from build123d import *

# Parameters (mm, degrees)
F1_DEPTH  = 25
F2_R      = 7.65
F3_DEPTH  = 1
F5_DEPTH  = 11
F7_W      = 10
F7_H      = 20
F10_W     = 10
F10_H     = 11
F13_START = -10
F13_DEPTH = 14
F14_START = -34
F14_DEPTH = 14
F15_R     = 5
F16_DEPTH = 7


with BuildPart() as f1:
    # F0 (on Top) → F1 (new body)
    with BuildSketch(Plane.XY):
        with BuildLine():
            ThreePointArc((0, 2), (0.5857864376, 0.5857864376), (2, 0))
            Line((2, 0), (116, 0))
            ThreePointArc((116, 0), (117.4142135624, 0.5857864376), (118, 2))
            Line((118, 2), (118, 98))
            ThreePointArc((118, 98), (117.4142135624, 99.4142135624), (116, 100))
            Line((116, 100), (2, 100))
            ThreePointArc((2, 100), (0.5857864376, 99.4142135624), (0, 98))
            Line((0, 98), (0, 2))
        make_face()
    extrude(amount=F1_DEPTH)

    # F2 (on face) → F3 (join)
    with BuildSketch(Plane.XY.offset(25)):
        with Locations((35, 28)):
            Circle(F2_R)
        with BuildLine():
            Line((23.7, 25.7), (23.7, 30.3))
            ThreePointArc((23.7, 30.3), (15, 39), (6.3, 30.3))
            Line((6.3, 30.3), (6.3, 25.7))
            ThreePointArc((6.3, 25.7), (15, 17), (23.7, 25.7))
        make_face()
        with Locations((53, 28)):
            Circle(F2_R)
    extrude(amount=F3_DEPTH)

    # F4 (on face) → F5 (cut)
    with BuildSketch(Plane.XY.offset(26)):
        Polygon((20.75, 25), (20.75, 31), (18.5, 31), (18.5, 34), (11.5, 34), (11.5, 31), (9.25, 31), (9.25, 25), (11.5, 25), (11.5, 22), (18.5, 22), (18.5, 25), align=None)
    extrude(amount=-F5_DEPTH, mode=Mode.SUBTRACT)

    # F7 (on offset) → F8 (revolve, cut)
    with BuildSketch(Plane.XY.offset(30)):
        with Locations((15, 80)):
            Rectangle(F7_W, F7_H)
        with Locations((35, 80)):
            Rectangle(F7_W, F7_H)
    revolve(axis=Axis((25, 70, 30), (1, 0, 0)), mode=Mode.SUBTRACT)

    # F10 (on offset) → F11 (revolve, cut)
    with BuildSketch(Plane.XY.offset(27)):
        with Locations((55, 55.5)):
            Rectangle(F10_W, F10_H)
    revolve(axis=Axis((55, 61, 27), (1, 0, 0)), mode=Mode.SUBTRACT)

    # F12 (on face) → F13 (cut)
    with BuildSketch(Plane.YZ.offset(118).offset(F13_START)):
        with BuildLine():
            Line((42, 1), (57, 1))
            ThreePointArc((57, 1), (92.8019763155, 40.7707415594), (49.5, 72.2100837829))
            ThreePointArc((49.5, 72.2100837829), (6.1980236845, 40.7707415594), (42, 1))
        make_face()
    extrude(amount=-F13_DEPTH, mode=Mode.SUBTRACT)

    # F12 (on face) → F14 (cut)
    with BuildSketch(Plane.YZ.offset(118).offset(F14_START)):
        with BuildLine():
            Line((42, 1), (57, 1))
            ThreePointArc((57, 1), (77.7846096908, 7.6061230866), (90.941125497, 25))
            Line((90.941125497, 25), (8.058874503, 25))
            ThreePointArc((8.058874503, 25), (21.2153903092, 7.6061230866), (42, 1))
        make_face()
    extrude(amount=-F14_DEPTH, mode=Mode.SUBTRACT)

    # F15 (on face) → F16 (cut)
    with BuildSketch(Plane.XY.offset(26)):
        with Locations((35, 28)):
            Circle(F15_R)
        with Locations((53, 28)):
            Circle(F15_R)
    extrude(amount=-F16_DEPTH, mode=Mode.SUBTRACT)


solid = f1.part
For this review, take the finished solid that the model builds, in its own axes (mm). A direction names the side the tool comes from. Give positions to 0.01 mm unless a question says otherwise; leave off trailing zeros. Order: outer loops, then holes, each group sorted by start corner. A loop starts at its lowest first (then second) coordinate and runs counter-clockwise, first axis right, second up. Notation, with made-up numbers: M 87.25,-6 L 135.25,-6 A19 cw 135.25,0 Z; hole C -23,-10 d6. An arc over 180 degrees is marked long. Answer in a Markdown table with one row per item. Add a question column.
(1) Consider section B-B on y = 55. State the section outline as (x, z) points.
(2) Consider section D-D on x = 96. State the section outline as (y, z) points.
(3) Consider section A-A on x = 35. State the section outline as (y, z) points, and give its area (3 significant figures).
(4) For faces 1 (the face through (77.1, 20.96, 7.79)), 2 (the face through (15.191, 38.998, 25.493)), 3 (the face through (60, 100, 12)), list the 3-axis set-ups (+Z, -Z, +X, -X, +Y, -Y) from which the entire face can be reached by the end or side of a thin tool; tool diameter is ignored.
(5) For pin 1 (5 mm diameter, centred on x = 95.5, y = 24.5, fed in from +Z); pin 2 (4 mm diameter, centred on x = 101.5, y = 49, fed in from +Z); pin 3 (2 mm diameter, centred on x = 104, y = 37.5, fed in from +Z), all flat-tipped, find the tip position at first contact; note any pin that passes through.
(6) Wall thickness on probe 1 along X at (y, z) = (29, 18.5); probe 2 along X at (y, z) = (59, 16.75); probe 3 along X at (y, z) = (40.5, 20.5): over which ranges is each line inside the solid? List them lowest first. Write a range as [from, to].
(7) Consider section C-C on z = 7.25. State the section outline as (x, y) points.
(8) Mouldability with a two-part tool opening along X and no side actions: class faces 4 (the face through (9, 28, 26)), 5 (the face through (53, 28, 19)), 6 (the face through (14.809, 17.002, 25.493)) as +X half, -X half, draft (parallel to the pull), parting line (faces both ways), or undercut.
Evaluation:
| question | item | result |
|---|---|---|
| 1 | outline | M 0,0 L 118,0 L 118,25 L 108,25 L 108,1 L 94,1 L 94,25 L 84,25 L 84,1 L 70,1 L 70,25 L 60,25 L 60,17.78 L 50,17.78 L 50,25 L 40,25 L 40,16.77 L 30,16.77 L 30,25 L 20,25 L 20,16.77 L 10,16.77 L 10,25 L 0,25 Z |
| 2 | outline | M 0,0 L 100,0 L 100,25 L 90.94,25 A36 cw 57,1 L 42,1 A36 cw 8.06,25 L 0,25 Z |
| 3 | outline | M 0,0 L 100,0 L 100,25 L 89.36,25 A20 cw 50.64,25 L 35.65,25 L 35.65,26 L 33,26 L 33,19 L 23,19 L 23,26 L 20.35,26 L 20.35,25 L 0,25 Z |
| 3 | area | 2,010 mm^2 |
| 4 | face 1 | +Z |
| 4 | face 2 | +Z, +Y |
| 4 | face 3 | +Z, -Z, +X, -X, +Y |
| 5 | pin 1 | stops at z = 25 |
| 5 | pin 2 | stops at z = 1 |
| 5 | pin 3 | stops at z = 1.42 |
| 6 | probe 1 | x = [0, 9.25], [20.75, 70], [84, 94], [108, 118] |
| 6 | probe 2 | x = [0, 10], [20, 30], [40, 50], [60, 70], [84, 94], [108, 118] |
| 6 | probe 3 | x = [0, 70], [84, 94], [108, 118] |
| 7 | outline | M 0,2 A2 ccw 2,0 L 116,0 A2 ccw 118,2 L 118,98 A2 ccw 116,100 L 2,100 A2 ccw 0,98 Z; hole M 70,21.73 L 84,21.73 L 84,77.27 L 70,77.27 Z; hole M 94,21.73 L 108,21.73 L 108,77.27 L 94,77.27 Z |
| 8 | face 4 | draft |
| 8 | face 5 | undercut |
| 8 | face 6 | undercut |
